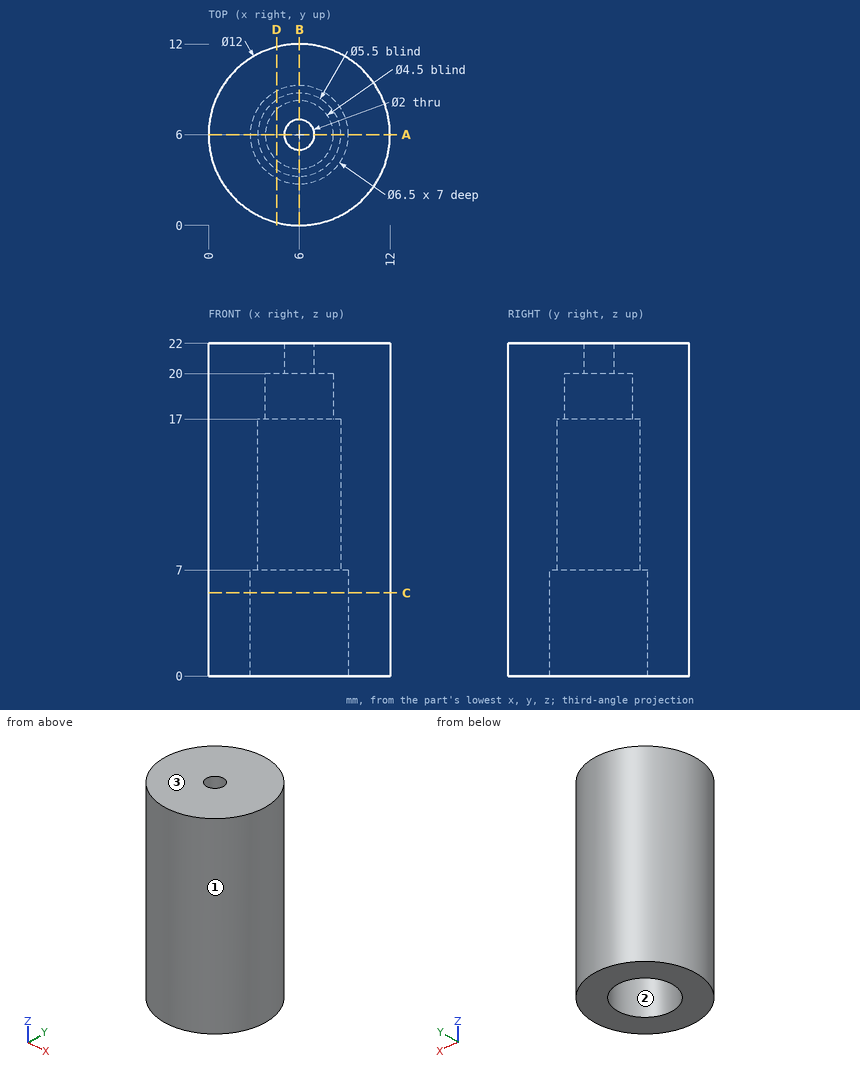
Study the drawing (mm; zero at the part's minimum x, y, z) and answer. Round coordinates to 2 decimals unless told otherwise and drop trailing zeros. Write each loop counter-clockwise with the first axis right and the second up, starting at its lowest first coordinate (ties: lowest second). Pieces come first, ordered by that corner, then holes. Notation, with made-up numbers: (65.5, 46) - (105.5, 46) arc R26 ccw to (105.5, 71) - close; hole circle Ø2 at (-1, 36.25). An arc over 180 degrees is marked (long way). Use a Markdown table: item, result. Add a question column.
1. For a pull along Y with two mould halves and no side action, classify the marked faces 1, 2 and 3 as +Y half, -Y half, draft (parallel to the pull), parting line (faces both ways), or undercut.
2. The part is cut by section D-D (x = 4.5). Write down the section's boundary in (y, z), and give its area (3 significant figures).
3. Consider line 1 (Y direction, x = 6, z = 18.8); line 2 (Y direction, x = 6, z = 3); line 3 (Z direction, x = 3.5, y = 6.5). Determine where each line is inside the solid, lowest interval first.
4. The part is cut by section A-A (y = 6). Write down the section's boundary in (x, z), and give its area (3 significant figures).
5. The part is cut by section C-C (z = 5.5). Write down the section's boundary in (x, y).
6. Flat-ended cylindrical pins translate along their axes: P1, Ø5, axis at x = 6, y = 6, coming from the -Z side; P2, Ø1.8, axis at x = 6, y = 6, coming from the -Z side. Find the tip coordinate at first contact, or state that the pin passes through.
Reported:
| question | item | result |
|---|---|---|
| 1 | face 1 | parting line |
| 1 | face 2 | undercut |
| 1 | face 3 | draft |
| 2 | outline | (0.19, 0) - (3.12, 0) - (3.12, 7) - (3.7, 7) - (3.7, 17) - (4.32, 17) - (4.32, 20) - (7.68, 20) - (7.68, 17) - (8.3, 17) - (8.3, 7) - (8.88, 7) - (8.88, 0) - (11.81, 0) - (11.81, 22) - (0.19, 22) - close |
| 2 | area | 159 mm^2 |
| 3 | line 1 | 0 to 3.75, 8.25 to 12 |
| 3 | line 2 | 0 to 2.75, 9.25 to 12 |
| 3 | line 3 | 17 to 22 |
| 4 | outline | (0, 0) - (2.75, 0) - (2.75, 7) - (3.25, 7) - (3.25, 17) - (3.75, 17) - (3.75, 20) - (5, 20) - (5, 22) - (0, 22) - close; (7, 20) - (8.25, 20) - (8.25, 17) - (8.75, 17) - (8.75, 7) - (9.25, 7) - (9.25, 0) - (12, 0) - (12, 22) - (7, 22) - close |
| 4 | area | 146 mm^2 |
| 5 | outline | circle Ø12 at (6, 6); hole circle Ø6.5 at (6, 6) |
| 6 | P1 | z = 17 |
| 6 | P2 | through |
